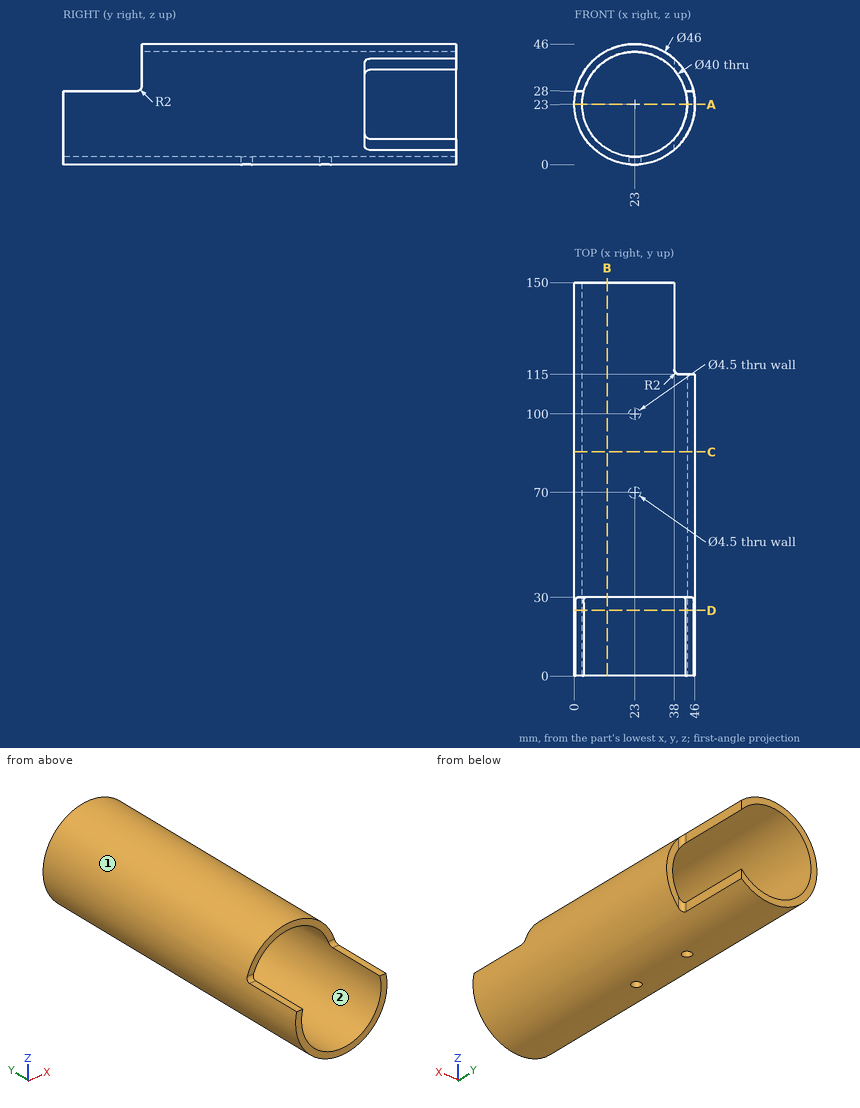
Job drawing, mm, ordinate dimensions from the low corner. One solid piece. Round coordinates to 2 decimals unless told otherwise and drop trailing zeros. Loops run counter-clockwise (first coordinate to the right, second up) from the corner with the lowest first, then second, coordinate; pieces in that order, holes last. Notation, with made-up numbers: (-5.75, -8.5) -> (25.25, -8.5) arc R5 cw to (25.25, -2.5) -> close; hole circle Ø8 at (74.25, 11.5). An arc over 180 degrees is marked (long way). Use CSV: the item, a comma, the result in double quotes. Start each with the question number.
Q1. Saw through at C-C on y = 85.5. Give the cut face in (x, z), and give its area (3 significant figures).
Q2. Flat gauge pins, fed straight in: pin 1 Ø10 at (y, z) = (98.5, 14) entering from +X; pin 2 Ø1.5 at (x, y) = (18.5, 69) entering from +Z; pin 3 Ø3.5 at (y, z) = (138.5, 8.5) entering from +X; pin 4 Ø12 at (x, z) = (26.5, 35.5) entering from -Y. Where does each tip first touch, or does it go through?
Q3. Saw through at D-D on y = 25. Give the cut face in (x, z), and give its area (3 significant figures).
Q4. Mould opens along Z. For the marked faces 1 and 2 say: +Z half, -Z half, draft (parallel to the pull), parting line (faces both ways), or undercut.
Q5. Saw through at A-A on z = 23. Give the cut face in (x, y).
Q6. Saw through at B-B on x = 12.5. Give the cut face in (y, z).
Q7. Drill centre lines: L1, parallel to Z at x = 23, y = 86; L2, parallel to X at y = 8, z = 22.5; L3, parallel to Z at x = 40, y = 43. Where is each one in solid material? Low to high.
Solutions:
1,outline,"circle Ø46 at (23, 23); hole circle Ø40 at (23, 23)"
1,area,"405 mm^2"
2,pin 1,"stops at x = 45.65"
2,pin 2,"stops at z = 45.69"
2,pin 3,"stops at x = 38"
2,pin 4,"passes through"
3,outline,"(0.55, 28) arc R23 ccw (long way) to (45.45, 28) -> (42.36, 28) arc R20 cw (long way) to (3.64, 28) -> close"
3,area,"233 mm^2"
4,face 1,"parting line"
4,face 2,"undercut"
5,outline,"(0, 0) -> (3, 0) -> (3, 150) -> (0, 150) -> close; (43, 0) -> (46, 0) -> (46, 115) -> (43, 115) -> close"
6,outline,"(0, 2.54) -> (150, 2.54) -> (150, 5.98) -> (0, 5.98) -> close; (30, 40.02) -> (150, 40.02) -> (150, 43.46) -> (30, 43.46) -> close"
7,L1,"z = 0 to 3, 43 to 46"
7,L2,"x = 0.01 to 3.01, 42.99 to 45.99"
7,L3,"z = 7.51 to 12.46, 33.54 to 38.49"
